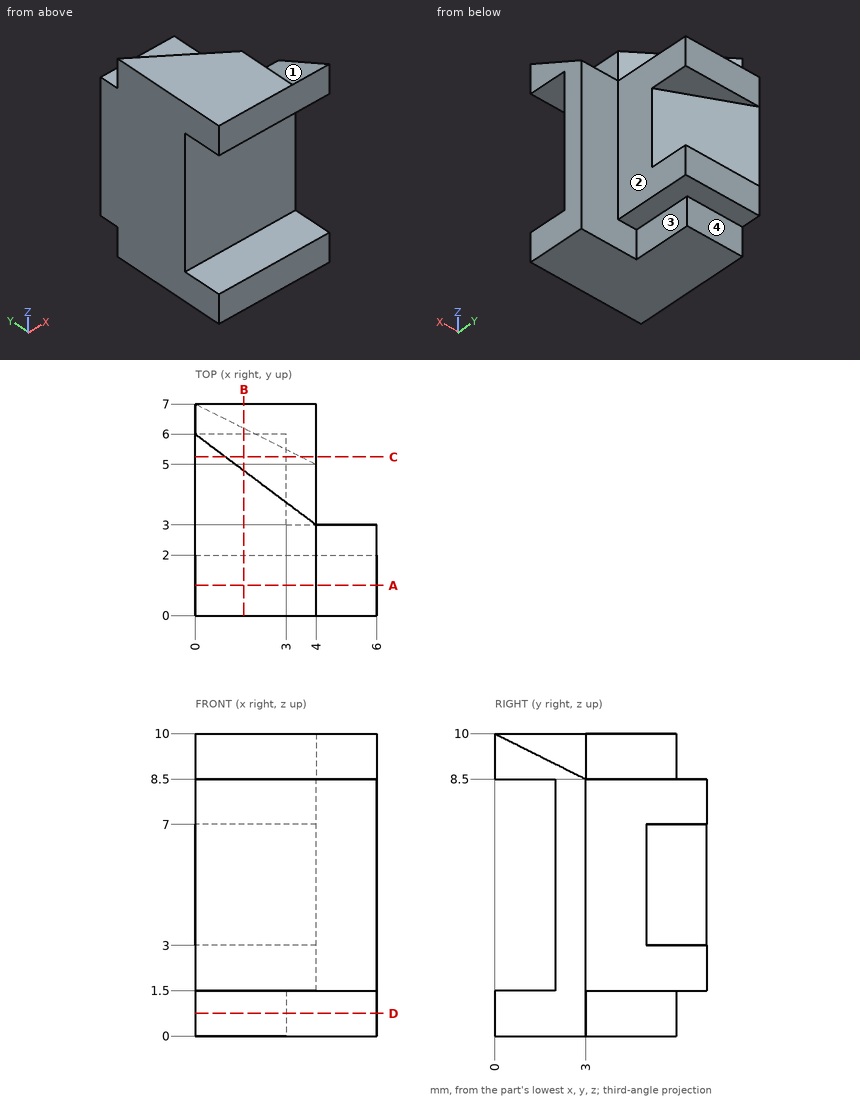
Here's the drawing with two shaded views (mm, measured from the low corner). I have some questions. A direction names the side the tool comes from. Give positions to 0.01 mm unless a question says otherwise; leave off trailing zeros. Loops run counter-clockwise (first coordinate to the right, second up) from the corner with the lowest first, then second, coordinate; pieces in that order, holes last. Notation, with made-up numbers: M 5,-14.75 L 18,-14.75 A27 cw 18,18.25 Z; hole C -1,-21.75 d2. An arc over 180 degrees is marked long. Use one line per item in the form item = value. Start each with the question number.
Q1. If we section it at C-C (y = 5.25): Write out the boundary of the cut face in (x, z), then the cut area to 3 significant figures.
Q2. Which directions (+Z, -Z, +X, -X, +Y, -Y) give clear straight access to the entire face, cutting with the end or side of a thin tool? Please do the marked faces 1, 2, 3 and 4.
Q3. If we section it at B-B (x = 1.6): Write out the boundary of the cut face in (y, z), then the cut area to 3 significant figures.
Q4. I need wall thicknesses on line 1 along Z through (x, y) = (2.55, 0.5); line 2 along Y through (x, z) = (3.8, 1); line 3 along Y through (x, z) = (5.6, 7). Which ranges of each line are inside material? Lowest first, please.
Q5. If we section it at A-A (y = 1): Write out the boundary of the cut face in (x, z), then the cut area to 3 significant figures.
Q6. Will these pins go through, and if not, where does the flat tip stop? pin 1 Ø2.5 at (x, z) = (4.5, 2.5) entering from +Y; pin 2 Ø1 at (x, z) = (2, 3) entering from -Y; pin 3 Ø1.2 at (y, z) = (4, 0.5) entering from +X; pin 4 Ø1.6 at (x, y) = (2.5, 6.5) entering from +Z.
Q7. If we section it at D-D (z = 0.75): Write out the boundary of the cut face in (x, y), then the cut area to 3 significant figures.
Taken from the geometry:
q1.outline = M 0,0 L 3,0 L 3,1.5 L 4,1.5 L 4,3 L 3.5,3 L 3.5,7 L 4,7 L 4,8.5 L 1,8.5 L 1,10 L 0,10 Z
q1.area = 32.0 mm^2
q2.face_1 = +Z, +X, +Y
q2.face_2 = +Z, -Z, +X, +Y
q2.face_3 = -Z, +X, +Y
q2.face_4 = -Z, +X, -X, +Y
q3.outline = M 0,0 L 6,0 L 6,1.5 L 7,1.5 L 7,3 L 6.2,3 L 6.2,7 L 7,7 L 7,8.5 L 4.8,8.5 L 4.8,10 L 0,10 L 0,8.5 L 2,8.5 L 2,1.5 L 0,1.5 Z
q3.area = 48.0 mm^2
q4.line_1 = 0 to 1.5, 8.5 to 10
q4.line_2 = 0 to 3
q4.line_3 = 2 to 3
q5.outline = M 0,0 L 6,0 L 6,1.5 L 0,1.5 Z; M 0,8.5 L 6,8.5 L 6,9.5 L 4,9.5 L 4,10 L 0,10 Z
q5.area = 17.0 mm^2
q6.pin_1 = 7
q6.pin_2 = 2
q6.pin_3 = 3
q6.pin_4 = 8.5
q7.outline = M 0,0 L 6,0 L 6,3 L 3,3 L 3,6 L 0,6 Z
q7.area = 27.0 mm^2
